Geometry check sheet. Reference: the model listing, model coordinates, mm. A direction names the side the tool comes from. Give positions to 0.01 mm unless a question says otherwise; leave off trailing zeros. Loops run counter-clockwise (first coordinate to the right, second up) from the corner with the lowest first, then second, coordinate; pieces in that order, holes last. Notation, with made-up numbers: (12, -34.75) - (24, -34.75) arc R7 ccw to (24, -22.75) - close; hole circle Ø2 at (70.5, 9.5). An arc over 180 degrees is marked (long way). Use a Markdown table: item, result. Add a question column.
1. Material ranges on L1, parallel to X at y = 126, z = 0; L2, parallel to Y at x = 24.5, z = 23.5; L3, parallel to Y at x = -2, z = 13.5, recorded low to high.
2. Depth check by flat-ended pin: P1, Ø8, axis at x = 50.5, z = 36.5, coming from the +Y side; P2, Ø5, axis at x = 17.5, y = 143.5, coming from the +Z side; P3, Ø6, axis at y = 195.5, z = -22, coming from the -X side. Enter the tip coordinate at first touch or a pass-through.
3. Cross-section at A-A on x = 0. Enter the section's corners in (y, z) (3 decimals), and give its area (3 significant figures).
4. Set-up check for faces 5 (the cylindrical face through (-2.06, 383.86, 9.3)), 6 (the cylindrical face through (-7.3, 190.7, -55.4)), 7 (the flat face through (1, 0, -1)): record each of +Z, -Z, +X, -X, +Y, -Y from which the full face is reachable in a straight line by a thin tool's end or side.
5. Cross-section at C-C on y = 350. Enter the section's corners in (x, z).
6. Draft check along X on faces 1 (the flat face through (15, 400.05, 17)), 2 (the flat face through (-1, 25.4, -1)), 3 (the cylindrical face through (-46.367, 184.702, -60.47)), 4 (the flat face through (12, 360.68, -1)). Enter one of: pulls with the +X half, pulls with the -X half, needs draft (parallel to the pull), parting line crosses it, or undercut.
7. Cross-section at B-B on z = 0. Enter the section's corners in (x, y) (3 decimals), and give its area (3 significant figures).
from build123d import *

# Parameters (mm, degrees)
SKETCH1_R           = 76.2
BOSS_EXTRUDE1_DEPTH = 381
FILLET1_R           = 6.35
SHELL4_START        = 25.4
SHELL4_OUTLINE_R    = 55.88
SHELL4_DEPTH        = 335.28
SKETCH3_R           = 9.525
CUT_EXTRUDE1_DEPTH  = 20.32


# Read off the part's stored shape, not the designer's step: Shell4
with BuildPart() as part:
    # Sketch1 → Boss-Extrude1 (new body)
    with BuildSketch(Plane(origin=(0, 0, 0), x_dir=(1, 0, 0), z_dir=(0, 1, 0))):
        with Locations(Location((0, 0, 0), (0, 0, 270))):
            Circle(SKETCH1_R)
    extrude(amount=BOSS_EXTRUDE1_DEPTH)

    # Fillet1
    fillet1_edges = [part.edges().sort_by_distance(p)[0] for p in [
        (0, 381, -76.2),
    ]]
    fillet(fillet1_edges, radius=FILLET1_R)

    # Sketch2 → Revolve1 (revolve)
    with BuildSketch(Plane.XY, mode=Mode.PRIVATE) as revolve1_sk:
        Polygon((-9.525, 381), (-9.525, 406.4), (-28.575, 406.4), (-28.575, 400.05), (-22.225, 400.05), (-22.225, 381), align=None)
    revolve(revolve1_sk.sketch.rotate(Axis((0, -1000, 0), (0, 1, 0)), 180), axis=Axis((0, -1000, 0), (0, 1, 0)))

    # Shell4 outline → Shell4 (cut)
    with BuildSketch(Plane(origin=(0, 0, 0), x_dir=(1, 0, 0), z_dir=(0, 1, 0)).offset(SHELL4_START)):
        Circle(SHELL4_OUTLINE_R)
    extrude(amount=SHELL4_DEPTH, mode=Mode.SUBTRACT)

    # Sketch3 → Cut-Extrude1 (cut)
    with BuildSketch(Plane(origin=(0, 381, 0), x_dir=(1, 0, 0), z_dir=(0, 1, 0))):
        Circle(SKETCH3_R)
    extrude(amount=-CUT_EXTRUDE1_DEPTH, mode=Mode.SUBTRACT)


solid = part.part
Values found:
| question | item | result |
|---|---|---|
| 1 | L1 | x = -76.2 to -55.88, 55.88 to 76.2 |
| 1 | L2 | y = 0 to 25.4, 360.68 to 381 |
| 1 | L3 | y = 0 to 25.4, 360.68 to 406.4 |
| 2 | P1 | stops at y = 381 |
| 2 | P2 | stops at z = 74.71 |
| 2 | P3 | stops at x = -73.79 |
| 3 | outline | (0, -76.2) - (374.65, -76.2) arc R6.35 ccw to (381, -69.85) - (381, -22.225) - (400.05, -22.225) - (400.05, -28.575) - (406.4, -28.575) - (406.4, -9.525) - (360.68, -9.525) - (360.68, -55.88) - (25.4, -55.88) - (25.4, 55.88) - (360.68, 55.88) - (360.68, 9.525) - (406.4, 9.525) - (406.4, 28.575) - (400.05, 28.575) - (400.05, 22.225) - (381, 22.225) - (381, 69.85) arc R6.35 ccw to (374.65, 76.2) - (0, 76.2) - close |
| 3 | area | 20,900 mm2 |
| 4 | face 5 | +Y |
| 4 | face 6 | none |
| 4 | face 7 | +Z, -Z, +X, -X, -Y |
| 5 | outline | circle Ø152.4 at (0, 0); hole circle Ø111.76 at (0, 0) |
| 6 | face 1 | needs draft |
| 6 | face 2 | undercut |
| 6 | face 3 | parting line crosses it |
| 6 | face 4 | undercut |
| 7 | outline | (-76.2, 0) - (76.2, 0) - (76.2, 374.65) arc R6.35 ccw to (69.85, 381) - (22.225, 381) - (22.225, 400.05) - (28.575, 400.05) - (28.575, 406.4) - (9.525, 406.4) - (9.525, 360.68) - (55.88, 360.68) - (55.88, 25.4) - (-55.88, 25.4) - (-55.88, 360.68) - (-9.525, 360.68) - (-9.525, 406.4) - (-28.575, 406.4) - (-28.575, 400.05) - (-22.225, 400.05) - (-22.225, 381) - (-69.85, 381) arc R6.35 ccw to (-76.2, 374.65) - close |
| 7 | area | 20,900 mm2 |
